```python
from build123d import *

# Parameters (mm, degrees)
SKETCH1_R           = 250
SKETCH1_R_2         = 180
SKETCH1_R_3         = 12.5
BOSS_EXTRUDE2_DEPTH = 20
REVOLVE1_ANGLE      = 180


with BuildPart() as part:
    # Sketch1 → Boss-Extrude2 (new body)
    with BuildSketch(Plane.XY):
        Circle(SKETCH1_R)
        Circle(SKETCH1_R_2, mode=Mode.SUBTRACT)
        with Locations((0, 217.200097765)):
            Circle(SKETCH1_R_3, mode=Mode.SUBTRACT)
        with Locations((108.600048882, 188.100802369)):
            Circle(SKETCH1_R_3, mode=Mode.SUBTRACT)
        with Locations((188.100802369, 108.600048882)):
            Circle(SKETCH1_R_3, mode=Mode.SUBTRACT)
        with Locations((217.200097765, 0)):
            Circle(SKETCH1_R_3, mode=Mode.SUBTRACT)
        with Locations((188.100802369, -108.600048882)):
            Circle(SKETCH1_R_3, mode=Mode.SUBTRACT)
        with Locations((108.600048882, -188.100802369)):
            Circle(SKETCH1_R_3, mode=Mode.SUBTRACT)
        with Locations((0, -217.200097765)):
            Circle(SKETCH1_R_3, mode=Mode.SUBTRACT)
        with Locations((-108.600048882, -188.100802369)):
            Circle(SKETCH1_R_3, mode=Mode.SUBTRACT)
        with Locations((-188.100802369, -108.600048882)):
            Circle(SKETCH1_R_3, mode=Mode.SUBTRACT)
        with Locations((-217.200097765, 0)):
            Circle(SKETCH1_R_3, mode=Mode.SUBTRACT)
        with Locations((-188.100802369, 108.600048882)):
            Circle(SKETCH1_R_3, mode=Mode.SUBTRACT)
        with Locations((-108.600048882, 188.100802369)):
            Circle(SKETCH1_R_3, mode=Mode.SUBTRACT)
    extrude(amount=BOSS_EXTRUDE2_DEPTH)

    # Sketch2 → Revolve1 (revolve)
    with BuildSketch(Plane(origin=(0, 0, 0), x_dir=(-1, 0, 0), z_dir=(0, 0, -1))):
        with BuildLine():
            Line((0, 180), (0, 200))
            ThreePointArc((0, 200), (200, 0), (0, -200))
            Line((0, -200), (0, -180))
            ThreePointArc((0, -180), (180, 0), (0, 180))
        make_face()
    revolve(axis=Axis((0, 180, 0), (0, -1, 0)), revolution_arc=REVOLVE1_ANGLE)


solid = part.part
```
Can you work these out from the model? Positions are in its coordinate system, mm. A direction names the side the tool comes from. Coordinates: 2 decimals unless noted, no trailing zeros. Order: outer loops, then holes, each group sorted by start corner. A loop starts at its lowest first (then second) coordinate and runs counter-clockwise, first axis right, second up.
1. For faces 4 (the face through (-198.02, 100.994, 9.86)), 5 (the face through (83.06, -159.69, 9.86)), which set-ups out of +Z, -Z, +X, -X, +Y, -Y let a thin tool reach every point of the face, with its end or its side?
2. If we section it at C-C (y = -73): Please give me the cut outline in (x, z).
3. If we section it at D-D (z = -33.5): Please give me the cut outline in (x, y), then the cut area to 3 significant figures.
4. If we section it at A-A (x = 0): Please give me the cut outline in (y, z), then the cut area to 3 significant figures.
5. Thinking about a two-plate mould opening in X: for faces 1 (the face through (-249.76, 10.99, 9.86)), 2 (the face through (-229.688, 0.55, 9.86)), 3 (the face through (-168, -110, 0)), which applies, +X half, -X half, draft (parallel to the pull), parting line (faces both ways), or undercut?
6. I need wall thicknesses on line 1 (X direction, y = 87, z = -64.5); line 2 (X direction, y = 85.5, z = -120.5); line 3 (Z direction, x = 206, y = -68.5). Which ranges of each line are inside material? Lowest first, please.
7. I'm going to push flat-ended pins straight in: pin 1 (15 mm diameter, centred on x = -188.1, y = -108.6, fed in from +Z); pin 2 (2 mm diameter, centred on x = 172.5, z = -59, fed in from -Y); pin 3 (8 mm diameter, centred on y = -58.5, z = -131, fed in from +X); pin 4 (8 mm diameter, centred on x = -154.5, z = -23, fed in from -Y). Where does each tip first touch, or does it pass through?
Entries:
1. face 4: +Z, -Z
1. face 5: +Z
2. outline: (-239.1, 0) - (-186.2, 0) arc R186.2 ccw to (186.2, 0) - (239.1, 0) - (239.1, 20) - (164.53, 20) - (164.53, 0) arc R164.53 cw to (-164.53, 0) - (-164.53, 20) - (-239.1, 20) - close
3. outline: circle Ø394.35 at (0, 0); hole circle Ø353.71 at (0, 0)
3. area: 23,900 mm2
4. outline: (-250, 0) - (-229.7, 0) - (-229.7, 20) - (-250, 20) - close; (-204.7, 0) - (-200, 0) arc R200 ccw to (200, 0) - (204.7, 0) - (204.7, 20) - (180, 20) - (180, 0) arc R180 cw to (-180, 0) - (-180, 20) - (-204.7, 20) - close; (229.7, 0) - (250, 0) - (250, 20) - (229.7, 20) - close
4. area: 13,700 mm2
5. face 1: parting line
5. face 2: undercut
5. face 3: draft
6. line 1: x = -168.14 to -143.77, 143.77 to 168.14
6. line 2: x = -134.79 to -102.81, 102.81 to 134.79
6. line 3: z = 0 to 20
7. pin 1: passes through
7. pin 2: stops at y = -84.42
7. pin 3: stops at x = 143.35
7. pin 4: stops at y = -129.75
